Could you check a few things on this drawing? It's one solid part, dimensions in mm from its lowest x, y, z. A direction names the side the tool comes from. Give positions to 0.01 mm unless a question says otherwise; leave off trailing zeros. Loops run counter-clockwise (first coordinate to the right, second up) from the corner with the lowest first, then second, coordinate; pieces in that order, holes last.
Q1. For the marked faces 1, 2 and 3, which set-ups out of +Z, -Z, +X, -X, +Y, -Y let a thin tool reach every point of the face, with its end or its side?
Q2. Suppose I cut it at A-A (z = 4.2). List the corners of the cut face in (x, y) for me.
Q3. Suppose I cut it at C-C (x = 2.75). List the corners of the cut face in (y, z) for me, and give its area (3 significant figures).
Q4. Thinking about a two-plate mould opening in Y: for the marked faces 4, 5, 6 and 7, which applies, pulls with the +Y half, pulls with the -Y half, needs draft (parallel to the pull), parting line crosses it, or undercut?
Q5. Suppose I cut it at D-D (z = 1.05). List the corners of the cut face in (x, y) for me.
Q6. Suppose I cut it at B-B (y = 6). List the corners of the cut face in (x, z) for me.
Q7. I need wall thicknesses on probe 1 along Y at (x, z) = (6, 0.8); probe 2 along Z at (x, y) = (5, 9.75); probe 3 along Y at (x, z) = (2.25, 4.35) (1 decimal). Which ranges of each line are inside material? Lowest first, please.
Q8. I'm going to push flat-ended pins straight in: P1, Ø4, axis at x = 3, y = 6.5, coming from the -Z side; P2, Ø1.5, axis at x = 3, z = 1.5, coming from the -Y side; P3, Ø1.8, axis at x = 6.5, y = 4.5, coming from the -Z side; P4, Ø2, axis at x = 3.5, z = 1.5, coming from the -Y side. Where does each tip first touch, or does it pass through?
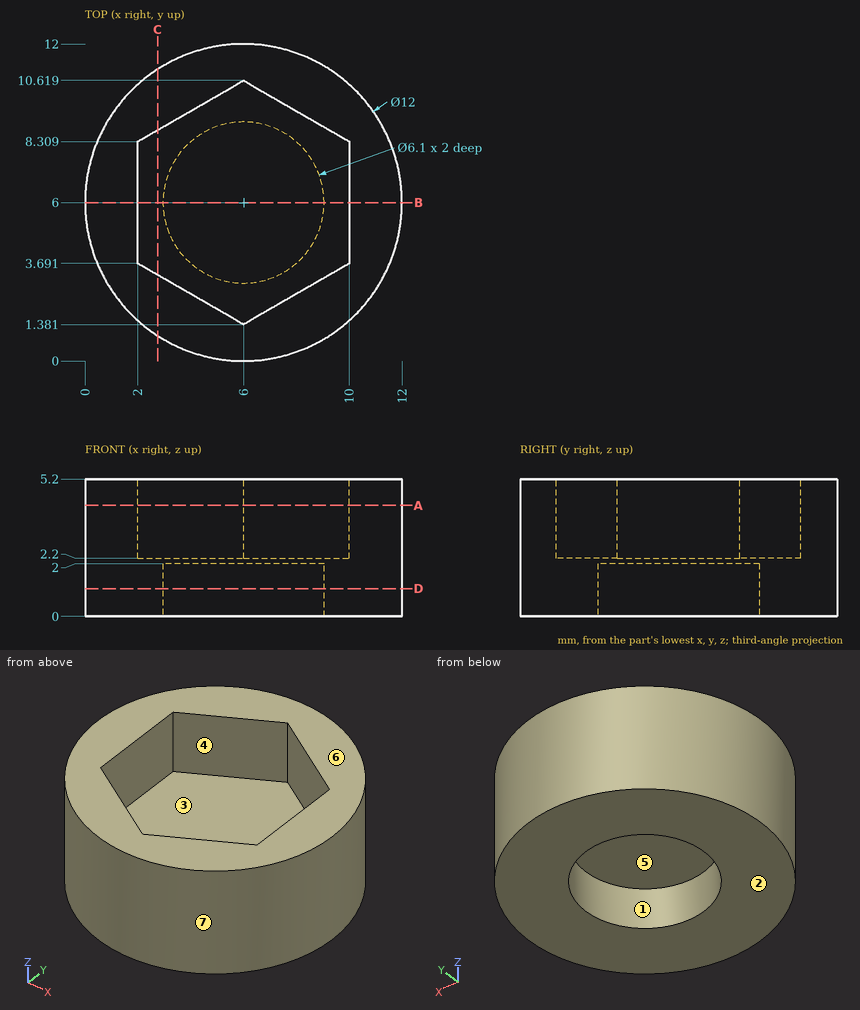
Solutions:
1. face 1: -Z
1. face 2: -Z, +X, -X, +Y, -Y
1. face 3: +Z
2. outline: circle Ø12 at (6, 6); hole (2, 3.69) - (6, 1.38) - (10, 3.69) - (10, 8.31) - (6, 10.62) - (2, 8.31) - close
3. outline: (0.96, 0) - (11.04, 0) - (11.04, 5.2) - (8.74, 5.2) - (8.74, 2.2) - (3.26, 2.2) - (3.26, 5.2) - (0.96, 5.2) - close
3. area: 36.0 mm2
4. face 4: undercut
4. face 5: undercut
4. face 6: needs draft
4. face 7: parting line crosses it
5. outline: circle Ø12 at (6, 6); hole circle Ø6.1 at (6, 6)
6. outline: (0, 0) - (2.95, 0) - (2.95, 2) - (9.05, 2) - (9.05, 0) - (12, 0) - (12, 5.2) - (10, 5.2) - (10, 2.2) - (2, 2.2) - (2, 5.2) - (0, 5.2) - close
7. probe 1: y = 0 to 2.95, 9.05 to 12
7. probe 2: z = 0 to 2.2
7. probe 3: y = 1.3 to 3.5, 8.5 to 10.7
8. P1: stops at z = 0
8. P2: stops at y = 0.44
8. P3: stops at z = 2
8. P4: stops at y = 0.19
